from build123d import *

# Parameters (mm, degrees)
SKETCH1_W           = 90
SKETCH1_H           = 24
SKETCH1_R           = 4
BOSS_EXTRUDE1_DEPTH = 9
SKETCH2_R           = 7.5
CUT_EXTRUDE3_DEPTH  = 52.788029505


with BuildPart() as part:
    # Sketch1 → Boss-Extrude1 (new, symmetric)
    with BuildSketch(Plane.XY):
        Rectangle(SKETCH1_W, SKETCH1_H)
        with Locations((-19, 0)):
            Circle(SKETCH1_R, mode=Mode.SUBTRACT)
        with Locations(Location((19, 0, 0), (0, 0, 180))):
            Circle(SKETCH1_R, mode=Mode.SUBTRACT)
    extrude(amount=BOSS_EXTRUDE1_DEPTH, both=True)

    # Sketch2 → Cut-Extrude3 (cut, through all)
    with BuildSketch(Plane(origin=(0, 12, 0), x_dir=(1, 0, 0), z_dir=(0, 1, 0))):
        with Locations(Location((-32.5, 0, 0), (0, 0, 270))):
            Circle(SKETCH2_R)
        with Locations(Location((32.5, 0, 0), (0, 0, 90))):
            Circle(SKETCH2_R)
    extrude(amount=-CUT_EXTRUDE3_DEPTH, mode=Mode.SUBTRACT)


solid = part.part
Source: CAD feature listing. Evaluate the final solid. Frame: model axes, mm. Round coordinates to 2 decimals unless told otherwise and drop trailing zeros. Order: outer loops, then holes, each group sorted by start corner. A loop starts at its lowest first (then second) coordinate and runs counter-clockwise, first axis right, second up. Notation, with made-up numbers: (54.25, 40.25) -> (60.25, 40.25) arc R26 cw to (60.25, 73.25) -> close; hole circle Ø6 at (-13, 38). An arc over 180 degrees is marked (long way). Answer as CSV lines item,"result".
Item 1: Pin query (flat end, axial travel): pin 1 Ø13 at (x, y) = (19, 0) entering from -Z; pin 2 Ø6.5 at (x, y) = (-19, 0) entering from +Z. Return the tip coordinate at first contact, or that it passes through.
A:
pin 1,"z = -9"
pin 2,"through"
Item 2: Section C-C, the plane y = -2.75. Return loops of the section in (x, z), plus the area to 3 significant figures.
A:
outline,"(-45, -9) -> (-21.9, -9) -> (-21.9, 9) -> (-45, 9) -> close; (-16.1, -9) -> (16.1, -9) -> (16.1, 9) -> (-16.1, 9) -> close; (21.9, -9) -> (45, -9) -> (45, 9) -> (21.9, 9) -> close; hole circle Ø15 at (-32.5, 0); hole circle Ø15 at (32.5, 0)"
area,"1,060 mm²"
Item 3: Pull-direction query (X, two-part tool) for faces 1 (the face through (-39.82, 0.17, -1.63)), 2 (the face through (-1, 0, -9)), 3 (the face through (-45, 0, 0)); classes: pulls with the +X half, pulls with the -X half, needs draft (parallel to the pull), parting line crosses it, or undercut.
A:
face 1,"undercut"
face 2,"needs draft"
face 3,"pulls with the -X half"
Item 4: Section B-B, the plane x = -32.5. Return loops of the section in (y, z).
A:
outline,"(-12, -9) -> (12, -9) -> (12, -7.5) -> (-12, -7.5) -> close; (-12, 7.5) -> (12, 7.5) -> (12, 9) -> (-12, 9) -> close"
Item 5: Section A-A, the plane z = 0. Return loops of the section in (x, y), plus the area to 3 significant figures.
A:
outline,"(-45, -12) -> (-40, -12) -> (-40, 12) -> (-45, 12) -> close; (-25, -12) -> (25, -12) -> (25, 12) -> (-25, 12) -> close; (40, -12) -> (45, -12) -> (45, 12) -> (40, 12) -> close; hole circle Ø8 at (-19, 0); hole circle Ø8 at (19, 0)"
area,"1,340 mm²"
Item 6: Section D-D, the plane y = 8.25. Return loops of the section in (x, z).
A:
outline,"(-45, -9) -> (45, -9) -> (45, 9) -> (-45, 9) -> close; hole circle Ø15 at (-32.5, 0); hole circle Ø15 at (32.5, 0)"
Item 7: Line query: L1, parallel to X at y = -4.75, z = 0; L2, parallel to X at y = -10.5, z = 3.25; L3, parallel to Y at x = -19, z = -3.25. Output: solid intervals per line, ascending.
A:
L1,"-45 to -40, -25 to 25, 40 to 45"
L2,"-45 to -39.26, -25.74 to 25.74, 39.26 to 45"
L3,"-12 to -4, 4 to 12"
